Input: part model. Units: mm. Frame: model coordinates. A direction names the side the tool comes from. Coordinates: 2 decimals unless noted, no trailing zeros. Write each loop counter-clockwise with the first axis right and the second up, starting at its lowest first coordinate (ties: lowest second). Pieces come first, ordered by that corner, then holes. Notation, with made-up numbers: (-17, 23.25) - (27, 23.25) arc R21 cw to (27, 36.25) - close; hole circle Ø6 at (19, 54). An arc over 180 degrees is marked (long way). Use CSV: the item, a comma, the result in double quotes.
```python
from build123d import *

# Parameters (mm, degrees)
F0_R           = 4.5
F1_DEPTH       = 5
F2_DEPTH       = 10
F4_D           = 3.2
F4_CBORE_D     = 5.6
F4_CBORE_DEPTH = 3
F5_T1_DEPTH    = 5
F6_R           = 1.5


# Not quite as in the source:
# - a fillet or chamfer that OpenCascade refuses, or shapes differently, is made with other operations: its cross-section is extruded or revolved along the edge and cut away or added
# - a feature names something its author has since deleted; it is built from what else it names


with BuildPart() as f1:
    # F0 (on Top) → F1 (new body)
    with BuildSketch(Plane.XY):
        with BuildLine():
            ThreePointArc((-12, -7.7459666924), (-5.1010205144, -6.3245553203), (-2, 0))
            ThreePointArc((-2, 0), (-4.3431457505, 5.6568542495), (-10, 8))
            ThreePointArc((-10, 8), (-17.9362375701, 1.0080343399), (-12, -7.7459666924))
        make_face()
        with Locations((-10, 0)):
            Circle(F0_R, mode=Mode.SUBTRACT)
        with BuildLine():
            ThreePointArc((-10, 8), (-4.3431457505, 5.6568542495), (-2, 0))
            ThreePointArc((-2, 0), (-5.1010205144, -6.3245553203), (-12, -7.7459666924))
            Line((-12, -7.7459666924), (-12, -15.5))
            ThreePointArc((-12, -15.5), (-6.5, -10), (-1, -15.5))
            ThreePointArc((-1, -15.5), (-1.5250628145, -17.8452078799), (-3, -19.7426406871))
            Line((-3, -19.7426406871), (-3, -21))
            Line((-3, -21), (18, -21))
            Line((18, -21), (18, -10))
            Line((18, -10), (18, 0))
            ThreePointArc((18, 0), (4.3431457505, -5.6568542495), (10, 8))
            Line((10, 8), (7, 8))
            Line((7, 8), (-10, 8))
        make_face()
        with BuildLine():
            Line((14.083025574, 44.3604283352), (7, 8))
            Line((7, 8), (10, 8))
            ThreePointArc((10, 8), (15.6568542495, 5.6568542495), (18, 0))
            Line((18, 0), (18, -10))
            Line((18, -10), (23, -10))
            Line((23, -10), (23, 43.5))
            ThreePointArc((23, 43.5), (22.2349698794, 40.9900199204), (20.2, 39.3334666688))
            Line((20.2, 39.3334666688), (20.2, 23.5))
            ThreePointArc((20.2, 23.5), (18.5, 21.8), (16.8, 23.5))
            Line((16.8, 23.5), (16.8, 39.3334666688))
            ThreePointArc((16.8, 39.3334666688), (14.5412211566, 41.3603574904), (14.083025574, 44.3604283352))
        make_face()
        with BuildLine():
            ThreePointArc((-1, -15.5), (-6.5, -10), (-12, -15.5))
            ThreePointArc((-12, -15.5), (-10.3890872965, -19.3890872965), (-6.5, -21))
            ThreePointArc((-6.5, -21), (-4.6405005753, -20.676124215), (-3, -19.7426406871))
            ThreePointArc((-3, -19.7426406871), (-1.5250628145, -17.8452078799), (-1, -15.5))
        make_face()
        with BuildLine():
            ThreePointArc((-6.5, -21), (-10.3890872965, -19.3890872965), (-12, -15.5))
            Line((-12, -15.5), (-12, -46.5))
            ThreePointArc((-12, -46.5), (-8.8452078799, -41.5250628145), (-3, -42.2573593129))
            Line((-3, -42.2573593129), (-3, -21))
            Line((-3, -21), (-6.5, -21))
        make_face()
        with BuildLine():
            ThreePointArc((23, 43.5), (18.9322123801, 47.9791955147), (14.083025574, 44.3604283352))
            ThreePointArc((14.083025574, 44.3604283352), (14.5412211566, 41.3603574904), (16.8, 39.3334666688))
            Line((16.8, 39.3334666688), (16.8, 43.5))
            ThreePointArc((16.8, 43.5), (18.5, 45.2), (20.2, 43.5))
            Line((20.2, 43.5), (20.2, 39.3334666688))
            ThreePointArc((20.2, 39.3334666688), (22.2349698794, 40.9900199204), (23, 43.5))
        make_face()
        with BuildLine():
            ThreePointArc((-3, -19.7426406871), (-4.6405005753, -20.676124215), (-6.5, -21))
            Line((-6.5, -21), (-3, -21))
            Line((-3, -21), (-3, -19.7426406871))
        make_face()
        with BuildLine():
            ThreePointArc((-3, -42.2573593129), (-8.8452078799, -41.5250628145), (-12, -46.5))
            ThreePointArc((-12, -46.5), (-6.5, -52), (-1, -46.5))
            ThreePointArc((-1, -46.5), (-1.5250628145, -44.1547921201), (-3, -42.2573593129))
        make_face()
        with BuildLine():
            Line((23, -10), (18, -10))
            Line((18, -10), (18, -21))
            Line((18, -21), (24.5, -21))
            ThreePointArc((24.5, -21), (19, -15.5), (24.5, -10))
            Line((24.5, -10), (23, -10))
        make_face()
        with BuildLine():
            ThreePointArc((30, -15.5), (28.3890872965, -11.6109127035), (24.5, -10))
            ThreePointArc((24.5, -10), (19, -15.5), (24.5, -21))
            ThreePointArc((24.5, -21), (28.3890872965, -19.3890872965), (30, -15.5))
        make_face()
        with BuildLine():
            ThreePointArc((18, 0), (15.6568542495, 5.6568542495), (10, 8))
            ThreePointArc((10, 8), (4.3431457505, -5.6568542495), (18, 0))
        make_face()
        with Locations((10, 0)):
            Circle(F0_R, mode=Mode.SUBTRACT)
    extrude(amount=-F1_DEPTH)

    # F0 (on Top) → F2 (join)
    with BuildSketch(Plane.XY):
        with BuildLine():
            ThreePointArc((30, -15.5), (28.3890872965, -11.6109127035), (24.5, -10))
            ThreePointArc((24.5, -10), (19, -15.5), (24.5, -21))
            ThreePointArc((24.5, -21), (28.3890872965, -19.3890872965), (30, -15.5))
        make_face()
        with BuildLine():
            ThreePointArc((-3, -42.2573593129), (-8.8452078799, -41.5250628145), (-12, -46.5))
            ThreePointArc((-12, -46.5), (-6.5, -52), (-1, -46.5))
            ThreePointArc((-1, -46.5), (-1.5250628145, -44.1547921201), (-3, -42.2573593129))
        make_face()
        with BuildLine():
            ThreePointArc((-12, -7.7459666924), (-5.1010205144, -6.3245553203), (-2, 0))
            ThreePointArc((-2, 0), (-4.3431457505, 5.6568542495), (-10, 8))
            ThreePointArc((-10, 8), (-17.9362375701, 1.0080343399), (-12, -7.7459666924))
        make_face()
        with Locations((-10, 0)):
            Circle(F0_R, mode=Mode.SUBTRACT)
        with BuildLine():
            ThreePointArc((-1, -15.5), (-6.5, -10), (-12, -15.5))
            ThreePointArc((-12, -15.5), (-10.3890872965, -19.3890872965), (-6.5, -21))
            ThreePointArc((-6.5, -21), (-4.6405005753, -20.676124215), (-3, -19.7426406871))
            ThreePointArc((-3, -19.7426406871), (-1.5250628145, -17.8452078799), (-1, -15.5))
        make_face()
        with BuildLine():
            ThreePointArc((-6.5, -21), (-10.3890872965, -19.3890872965), (-12, -15.5))
            Line((-12, -15.5), (-12, -46.5))
            ThreePointArc((-12, -46.5), (-8.8452078799, -41.5250628145), (-3, -42.2573593129))
            Line((-3, -42.2573593129), (-3, -21))
            Line((-3, -21), (-6.5, -21))
        make_face()
        with BuildLine():
            ThreePointArc((-3, -19.7426406871), (-4.6405005753, -20.676124215), (-6.5, -21))
            Line((-6.5, -21), (-3, -21))
            Line((-3, -21), (-3, -19.7426406871))
        make_face()
        with BuildLine():
            Line((23, -10), (18, -10))
            Line((18, -10), (18, -21))
            Line((18, -21), (24.5, -21))
            ThreePointArc((24.5, -21), (19, -15.5), (24.5, -10))
            Line((24.5, -10), (23, -10))
        make_face()
        with BuildLine():
            ThreePointArc((-10, 8), (-4.3431457505, 5.6568542495), (-2, 0))
            ThreePointArc((-2, 0), (-5.1010205144, -6.3245553203), (-12, -7.7459666924))
            Line((-12, -7.7459666924), (-12, -15.5))
            ThreePointArc((-12, -15.5), (-6.5, -10), (-1, -15.5))
            ThreePointArc((-1, -15.5), (-1.5250628145, -17.8452078799), (-3, -19.7426406871))
            Line((-3, -19.7426406871), (-3, -21))
            Line((-3, -21), (18, -21))
            Line((18, -21), (18, -10))
            Line((18, -10), (18, 0))
            ThreePointArc((18, 0), (4.3431457505, -5.6568542495), (10, 8))
            Line((10, 8), (7, 8))
            Line((7, 8), (-10, 8))
        make_face()
        with BuildLine():
            ThreePointArc((18, 0), (15.6568542495, 5.6568542495), (10, 8))
            ThreePointArc((10, 8), (4.3431457505, -5.6568542495), (18, 0))
        make_face()
        with Locations((10, 0)):
            Circle(F0_R, mode=Mode.SUBTRACT)
    extrude(amount=-F2_DEPTH)

    # F4 (through all)
    with Locations(Plane(origin=(0, 0, -10), x_dir=(1, 0, 0), z_dir=(0, 0, -1))):
        with Locations((-6.5, 46.5), (-6.5, 15.5), (24.5, 15.5)):
            CounterBoreHole(F4_D / 2, F4_CBORE_D / 2, F4_CBORE_DEPTH)

    # F5: fillet of radius 3 on 1 edges, made by hand

    # F5_s2 → F5_t1 (join)
    with BuildSketch(Plane.XY.offset(-5)):
        with BuildLine():
            ThreePointArc((25.4705882353, -10.0863174754), (23.6991050335, -9.0584665784), (23, -7.1333997347))
            Line((23, -7.1333997347), (22.7, -7.1333997347))
            Line((22.7, -7.1333997347), (22.7, -10))
            Line((22.7, -10), (23, -10.3))
            ThreePointArc((23, -10.3), (24.5, -10.3), (25.4176470588, -10.3816092494))
            Line((25.4176470588, -10.3816092494), (25.4705882353, -10.0863174754))
        make_face()
    extrude(amount=F5_T1_DEPTH)

    # F6
    f6_edges = [f1.edges().sort_by_distance(p)[0] for p in [
        (-3, -21, -5),
    ]]
    fillet(f6_edges, radius=F6_R)


solid = f1.part
```
(1) Reachability of faces 1 (the flat face through (-3, -33, -5)), 2 (the cylindrical face through (15.719, 5.594, -7.465)), 3 (the cylindrical face through (-5.208, -13.016, -8.521)) from +Z, -Z, +X, -X, +Y, -Y: full face, straight path, thin tool, end or side. Return the list, or none.
Check values:
face 1,"+Z, -Z, +X"
face 2,"-Z, +X, +Y"
face 3,"-Z"
(2) Cut plane D-D on x = -6.5. Return loops of the section in (y, z).
Check values:
outline,"(-52, -10) - (-49.3, -10) - (-49.3, -7) - (-48.1, -7) - (-48.1, 0) - (-52, 0) - close; (-44.9, -7) - (-43.7, -7) - (-43.7, -10) - (-18.3, -10) - (-18.3, -7) - (-17.1, -7) - (-17.1, 0) - (-44.9, 0) - close; (-13.9, -7) - (-12.7, -7) - (-12.7, -10) - (-2.83, -10) - (-2.83, 0) - (-13.9, 0) - close; (2.83, -10) - (8, -10) - (8, 0) - (2.83, 0) - close"
(3) Cut plane A-A on y = 33. Return loops of the section in (x, z), and give its area (4 significant figures).
Check values:
outline,"(11.87, -5) - (16.8, -5) - (16.8, 0) - (11.87, 0) - close; (20.2, -5) - (23, -5) - (23, 0) - (20.2, 0) - close"
area,"38.65 mm^2"
(4) Draft query along X for faces 4 (the flat face through (26, -14, -7)), 5 (the flat face through (0, -15, -10)), 6 (the cylindrical face through (30, -15.6, -4.9)). Return one class per face: pulls with the +X half, pulls with the -X half, needs draft (parallel to the pull), parting line crosses it, or undercut.
Check values:
face 4,"undercut"
face 5,"needs draft"
face 6,"pulls with the +X half"
(5) Ray query, probe 1 along X at (y, z) = (-15.5, -8.1); probe 2 along X at (y, z) = (-16, -6.25); probe 3 along Y at (x, z) = (-6.5, -2.25). Return the intervals inside material, ascending. Write a range as from..to.
Check values:
probe 1,"-12..-9.3, -3.7..21.7, 27.3..30"
probe 2,"-12..-8.02, -4.98..22.98, 26.02..29.98"
probe 3,"-52..-48.1, -44.9..-17.1, -13.9..-2.83, 2.83..8"
(6) Cut plane B-B on z = -8. Return loops of the section in (x, y).
Check values:
outline,"(-12, -46.5) arc R5.5 ccw (long way) to (-3, -42.26) - (-3, -22.5) arc R1.5 cw to (-1.5, -21) - (24.5, -21) arc R5.5 ccw to (24.5, -10) - (18, -10) - (18, 0) arc R8 ccw to (10, 8) - (-10, 8) arc R8 ccw to (-12, -7.75) - close; hole circle Ø9 at (-10, 0); hole circle Ø5.6 at (-6.5, -46.5); hole circle Ø5.6 at (-6.5, -15.5); hole circle Ø9 at (10, 0); hole circle Ø5.6 at (24.5, -15.5)"
(7) Cut plane C-C on z = -1. Return loops of the section in (x, y), and give its area (3 significant figures).
Check values:
outline,"(-12, -46.5) arc R5.5 ccw (long way) to (-3, -42.26) - (-3, -22.5) arc R1.5 cw to (-1.5, -21) - (24.5, -21) arc R5.5 ccw to (25.47, -10.09) arc R3 cw to (23, -7.13) - (23, 43.5) arc R4.5 ccw to (14.08, 44.36) - (7, 8) - (-10, 8) arc R8 ccw to (-12, -7.75) - close; hole circle Ø9 at (-10, 0); hole circle Ø3.2 at (-6.5, -46.5); hole circle Ø3.2 at (-6.5, -15.5); hole circle Ø9 at (10, 0); hole (16.8, 23.5) arc R1.7 ccw to (20.2, 23.5) - (20.2, 43.5) arc R1.7 ccw to (16.8, 43.5) - close; hole circle Ø3.2 at (24.5, -15.5)"
area,"1,680 mm^2"
(8) Pin query (flat end, axial travel): pin 1 Ø1 at (y, z) = (2.5, -1.5) entering from -X; pin 2 Ø1.5 at (y, z) = (-6.5, -6.5) entering from +X; pin 3 Ø9 at (x, y) = (-6.5, -46.5) entering from +Z; pin 4 Ø8 at (x, y) = (10, 0) entering from +Z. Return the tip coordinate at first contact, or that it passes through.
Check values:
pin 1,"x = -17.75"
pin 2,"x = 18"
pin 3,"z = 0"
pin 4,"through"
